```python
from build123d import *

# Parameters (mm, degrees)
F0_W           = 50.8
F0_H           = 50.8
F1_DEPTH       = 25.4
F3_D           = 5.5
F3_CBORE_D     = 9.75
F3_CBORE_DEPTH = 5
F4_R           = 5.08


with BuildPart() as f1:
    # F0 (on Top) → F1 (new body)
    with BuildSketch(Plane.XY):
        Rectangle(F0_W, F0_H)
    extrude(amount=F1_DEPTH)

    # F3 (through all)
    with Locations(Plane.XY.offset(25.4)):
        with Locations((0, 0)):
            CounterBoreHole(F3_D / 2, F3_CBORE_D / 2, F3_CBORE_DEPTH)

    # F4
    f4_edges = [f1.edges().sort_by_distance(p)[0] for p in [
        (-25.4, 0, 25.4),
        (0, 25.4, 25.4),
        (25.4, 0, 25.4),
        (0, -25.4, 25.4),
    ]]
    fillet(f4_edges, radius=F4_R)


solid = f1.part
```
Check sheet for the modelled part. Datum: model origin and axes. Units: mm. A direction names the side the tool comes from. Give positions to 0.01 mm unless a question says otherwise; leave off trailing zeros. Order: outer loops, then holes, each group sorted by start corner. A loop starts at its lowest first (then second) coordinate and runs counter-clockwise, first axis right, second up. Notation, with made-up numbers: M 40,87 L 48,87 A20 ccw 48,105 Z; hole C 24.25,69 d1. An arc over 180 degrees is marked long. Answer in a Markdown table with one row per item.
1) Thickness scan on L1, parallel to Y at x = 0, z = 10.75; L2, parallel to X at y = 0.5, z = 13.25; L3, parallel to Y at x = 0, z = 22.7 (3 decimals). Record the ranges inside material, lowest first. Write a range as [from, to].
Filled sheet:
| item | result |
|---|---|
| L1 | y = [-25.4, -2.75], [2.75, 25.4] |
| L2 | x = [-25.4, -2.7], [2.7, 25.4] |
| L3 | y = [-24.808, -4.875], [4.875, 24.808] |
2) Gauge pin test, flat ends, axial feed: P1, Ø9, axis at x = 0, y = 0, coming from the +Z side; P2, Ø8, axis at x = -0.5, y = -1, coming from the +Z side. Record the tip position at first contact, or that the pin passes through.
Filled sheet:
| item | result |
|---|---|
| P1 | stops at z = 20.4 |
| P2 | stops at z = 25.4 |
3) Release check for a two-part mould opening along X. For faces 3 (the cylindrical face through (0.596, -2.685, 10.057)), 4 (the flat face through (-25.4, 0, 10)), 5 (the cylindrical face through (-0.635, 4.834, 22.935)), 6 (the cylindrical face through (0.356, -23.951, 23.872)) record: +X half, -X half, draft (parallel to the pull), parting line (faces both ways), or undercut.
Filled sheet:
| item | result |
|---|---|
| face 3 | undercut |
| face 4 | -X half |
| face 5 | undercut |
| face 6 | draft |
4) Cross-section at A-A, the plane y = 0. Enter the section's corners in (x, z) (3 decimals).
Filled sheet:
| item | result |
|---|---|
| outline | M -25.4,0 L -2.75,0 L -2.75,20.4 L -4.875,20.4 L -4.875,25.4 L -20.32,25.4 A5.08 ccw -25.4,20.32 Z; M 2.75,0 L 25.4,0 L 25.4,20.32 A5.08 ccw 20.32,25.4 L 4.875,25.4 L 4.875,20.4 L 2.75,20.4 Z |
5) Access from +Z, -Z, +X, -X, +Y, -Y to the whole of each face (thin tool, end or side, straight path). Record for faces 1 (the flat face through (5, 0, 0)), 2 (the flat face through (2.1, -2.1, 20.4)).
Filled sheet:
| item | result |
|---|---|
| face 1 | -Z, +X, -X, +Y, -Y |
| face 2 | +Z |
